Autodesk Inventor part; units mm, degrees
ref_plane "YZ Plane" through (0, 0, 0) normal (1, 0, 0) x (0, 1, 0)
ref_plane "XZ Plane" through (0, 0, 0) normal (0, 1, 0) x (-1, 0, 0)
ref_plane "XY Plane" through (0, 0, 0) normal (0, 0, 1) x (1, 0, 0)
sketch "Skizze1" plane through (0, 0, 0) normal (0, 1, 0) x (-1, 0, 0)
  line L0 (0, 0) -> (140, 0)
  line L1 (140, 0) -> (140, 140)
  line L2 (140, 140) -> (0, 140)
  line L3 (0, 140) -> (0, 0)
  dimension "d0" = 140
  dimension "d1" = 140
extrude "Extrusion1" add sketch "Skizze1" along normal blind 18
sketch "Skizze2" plane through (0, 18, 0) normal (0, 1, 0) x (1, 0, 0)
  line L0 (0, 0) -> (-140, 0)
  line L1 (-140, 0) -> (-140, -140)
  line L2 (-140, -140) -> (0, -140)
  line L3 (0, -140) -> (0, 0)
  point P0 (-131, -15)
  point P1 (-131, -125)
  point P2 (-9, -15)
  point P3 (-9, -125)
  dimension "d4" = 15
  dimension "d5" = 15
  dimension "d6" = 15
  dimension "d7" = 15
  dimension "d8" = 9
  dimension "d9" = 9
  dimension "d10" = 9
  dimension "d11" = 9
hole "Bohrung1" at (-131, 18, 15) at (-131, 18, 125) at (-9, 18, 15) at (-9, 18, 125) direction (0, -1, 0) diameter 2 end through all countersink diameter 5 countersink angle 90
fillet "Rundung1" radius 5 4 edges at (-140, 9, 0) (-140, 9, 140) (0, 9, 140) (0, 9, 0)
sketch "Skizze3" plane through (0, 18, 0) normal (0, 1, 0) x (1, 0, 0)
  line L0 (-5, 0) -> (-135, 0)
  line L1 (-140, -5) -> (-140, -135)
  line L2 (0, -135) -> (0, -5)
  line L3 (-120, -45) -> (-20, -45)
  line L4 (-20, -45) -> (-20, -85)
  line L5 (-20, -85) -> (-120, -85)
  line L6 (-120, -85) -> (-120, -45)
  circle A0 centre (-70, -25) radius 2.5
  point P0 (0, 0)
  dimension "d20" = 20
  dimension "d23" = 100
  dimension "d24" = 40
  dimension "d25" = 45
  dimension "d26" = 5
  dimension "d27" = 70
  dimension "d28" = 25
extrude "Extrusion2" cut sketch "Skizze3" against normal blind 18
properties part number "Deckel" material "Eiche, weiß"
The listing builds one solid part. Answer for the finished solid, in the listing's coordinates (mm). A direction names the side the tool comes from. Give positions to 0.01 mm unless a question says otherwise; leave off trailing zeros. Order: outer loops, then holes, each group sorted by start corner. A loop starts at its lowest first (then second) coordinate and runs counter-clockwise, first axis right, second up. Notation, with made-up numbers: (37, 88) - (55, 88) arc R23 cw to (55, 121) - close; hole circle Ø1 at (26, -18). An arc over 180 degrees is marked (long way). One line per item, written item: value. Start each with the question number.
1) Given pin 1 Ø2.5 at (x, z) = (-9, 125) entering from +Y; pin 2 Ø1.6 at (x, z) = (-131, 125) entering from +Y, each flat-ended and moving along its own axis, determine where each tip first touches the part or whether it passes through.
2) A cutting plane is placed at D-D on y = 7.25. Give the vertices of the cut face in (x, z).
3) A cutting plane is placed at A-A on x = -26. Give the vertices of the cut face in (y, z), then the cut area to 3 significant figures.
4) A cutting plane is placed at C-C on x = -70. Give the vertices of the cut face in (y, z).
5) A tool of negligible diameter and unlimited length cuts with its end or side. For faces 1 (the face through (-71, 9, 140)), 2 (the face through (-20, 9, 65)), from which of +Z, -Z, +X, -X, +Y, -Y can it reach the whole face along a straight path? Write none if from no direction.
6) Find the intervals of material crossed by L1, parallel to Z at x = -9, y = 11.25; L2, parallel to X at y = 8.75, z = 15; L3, parallel to Z at x = -33.5, y = 11.75, in increasing order.
7) A cutting plane is placed at B-B on z = 74. Give the vertices of the cut face in (x, y), then the cut area to 3 significant figures.
Answer sheet:
1. pin 1: stops at y = 16.75
1. pin 2: passes through
2. outline: (-140, 5) arc R5 ccw to (-135, 0) - (-5, 0) arc R5 ccw to (0, 5) - (0, 135) arc R5 ccw to (-5, 140) - (-135, 140) arc R5 ccw to (-140, 135) - close; hole circle Ø2 at (-131, 15); hole circle Ø2 at (-131, 125); hole (-120, 45) - (-20, 45) - (-20, 85) - (-120, 85) - close; hole circle Ø5 at (-70, 25); hole circle Ø2 at (-9, 15); hole circle Ø2 at (-9, 125)
3. outline: (0, 0) - (18, 0) - (18, 45) - (0, 45) - close; (0, 85) - (18, 85) - (18, 140) - (0, 140) - close
3. area: 1,800 mm2
4. outline: (0, 0) - (18, 0) - (18, 22.5) - (0, 22.5) - close; (0, 27.5) - (18, 27.5) - (18, 45) - (0, 45) - close; (0, 85) - (18, 85) - (18, 140) - (0, 140) - close
5. face 1: +Z, +X, -X, +Y, -Y
5. face 2: +Y, -Y
6. L1: z = 0 to 14, 16 to 124, 126 to 140
6. L2: x = -140 to -132, -130 to -10, -8 to 0
6. L3: z = 0 to 45, 85 to 140
7. outline: (-140, 0) - (-120, 0) - (-120, 18) - (-140, 18) - close; (-20, 0) - (0, 0) - (0, 18) - (-20, 18) - close
7. area: 720 mm2
